For this review, take the finished solid that the model builds, in its own axes (mm). Face numbers are marked on the shaded views. A direction names the side the tool comes from. Give positions to 0.01 mm unless a question says otherwise; leave off trailing zeros. Order: outer loops, then holes, each group sorted by start corner. A loop starts at its lowest first (then second) coordinate and runs counter-clockwise, first axis right, second up. Notation, with made-up numbers: (39, 5) - (66, 5) arc R16 cw to (66, 26) - close; hole circle Ø2 at (-27.5, -30.5). An arc over 180 degrees is marked (long way). One line per item, written item: value.
```python
from build123d import *

# Parameters (mm, degrees)
SKETCH1_R           = 3.5
SKETCH1_R_2         = 4.5
BOSS_EXTRUDE1_DEPTH = 5
SKETCH2_R           = 8.75
SKETCH2_R_2         = 3.5
SKETCH2_R_3         = 4.5
BOSS_EXTRUDE2_DEPTH = 5


with BuildPart() as part:
    # Sketch1 → Boss-Extrude1 (new body)
    with BuildSketch(Plane.XY):
        with BuildLine():
            Line((-12.068862554, -6.04917818), (-9.828426191, -10.519127274))
            ThreePointArc((-9.828426191, -10.519127274), (-9.022245749, -17.239185417), (-12.680657026, -22.933492686))
            Line((-12.680657026, -22.933492686), (-18.627117662, -27.496435605))
            ThreePointArc((-18.627117662, -27.496435605), (-21.193595331, -47.96861112), (-0.691265287, -50.281886009))
            Line((-0.691265287, -50.281886009), (7.089345754, -44))
            Line((7.089345754, -44), (46.481655875, -37.054072893))
            Line((46.481655875, -37.054072893), (39.535728768, 2.338237227))
            ThreePointArc((39.535728768, 2.338237227), (23.15933572, 3.004735652), (8.554710295, 10.443511467))
            ThreePointArc((8.554710295, 10.443511467), (-8.431460103, 10.543267071), (-12.068862554, -6.04917818))
        make_face()
        Circle(SKETCH1_R, mode=Mode.SUBTRACT)
        with Locations((-9.8, -39)):
            Circle(SKETCH1_R_2, mode=Mode.SUBTRACT)
    extrude(amount=-BOSS_EXTRUDE1_DEPTH)

    # Sketch2 → Boss-Extrude2 (add)
    # profile 1 of 2: a face of its own
    with BuildSketch(Plane(origin=(0, 0, -5), x_dir=(-1, 0, 0), z_dir=(0, 0, -1))):
        with Locations(Location((0, 0, 0), (0, 0, 180))):
            Circle(SKETCH2_R)
        with Locations(Location((0, 0, 0), (0, 0, 180))):
            Circle(SKETCH2_R_2, mode=Mode.SUBTRACT)
    # profile 2 of 2: a face of its own
    with BuildSketch(Plane(origin=(0, 0, -5), x_dir=(-1, 0, 0), z_dir=(0, 0, -1))):
        with Locations(Location((9.8, -39, 0), (0, 0, 180))):
            Circle(SKETCH2_R)
        with Locations(Location((9.8, -39, 0), (0, 0, 180))):
            Circle(SKETCH2_R_3, mode=Mode.SUBTRACT)
    extrude(amount=BOSS_EXTRUDE2_DEPTH)


solid = part.part
```
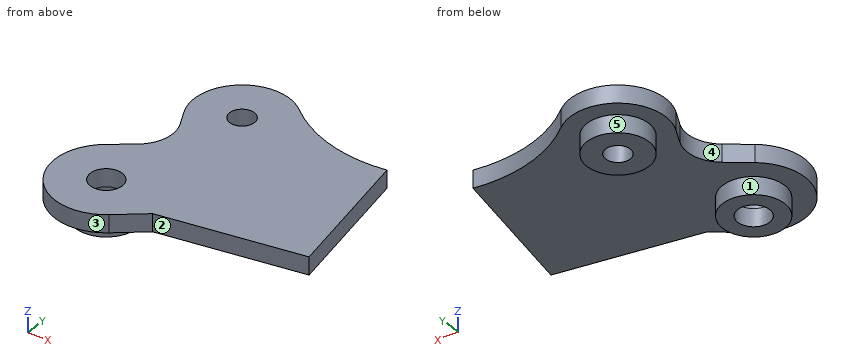
(1) Machinability: for the marked faces 4 and 5, which of the approach directions +Z, -Z, +X, -X, +Y, -Y give a long, thin tool a straight path to every point of the face, cutting with its end or side? Answer none if there is none.
Answers below:
face 4: +Z, -Z, -X
face 5: -Z
(2) Take a section at C-C (y = -5). Write out the cut boundary in (x, z), then the cut area to 3 significant figures.
Answers below:
outline: (-12.54, -5) - (-7.18, -5) - (-7.18, -10) - (7.18, -10) - (7.18, -5) - (40.83, -5) - (40.83, 0) - (-12.54, 0) - close
area: 339 mm^2
(3) Wall thickness on line 1 (X direction, y = -39, z = -8.9); line 2 (Y direction, x = 0, z = -6.8); line 3 (Z direction, x = 17.5, y = -38.5): over which ranges is each line inside the solid? List them lowest first. Write a range as from..to.
Answers below:
line 1: x = -18.55..-14.3, -5.3..-1.05
line 2: y = -8.75..-3.5, 3.5..8.75
line 3: z = -5..0
(4) Take a section at A-A (y = -39). Write out the cut boundary in (x, z), then the cut area to 3 significant figures.
Answers below:
outline: (-24.3, -5) - (-18.55, -5) - (-18.55, -10) - (-14.3, -10) - (-14.3, 0) - (-24.3, 0) - close; (-5.3, -10) - (-1.05, -10) - (-1.05, -5) - (35.45, -5) - (35.45, 0) - (-5.3, 0) - close
area: 296 mm^2
(5) Take a section at D-D (x = -4.5). Write out the cut boundary in (y, z), then the cut area to 3 significant figures.
Answers below:
outline: (-52.5, -5) - (-45.96, -5) - (-45.96, -10) - (-32.04, -10) - (-32.04, -5) - (-7.5, -5) - (-7.5, -10) - (7.5, -10) - (7.5, -5) - (12.73, -5) - (12.73, 0) - (-52.5, 0) - close
area: 471 mm^2
(6) For P1, Ø6, axis at x = 17.5, z = -7, coming from the -Y side; P2, Ø1, axis at x = 8.5, z = -2, coming from the -Y side; P3, Ø3, axis at y = 1, z = -2.5, coming from the +X side, all flat-tipped, find the tip position at first contact; note any pin that passes through.
Answers below:
P1: stops at y = -42.56
P2: stops at y = -43.84
P3: stops at x = 40.04
(7) Take a section at B-B (z = -6.25). Write out the cut boundary in (x, y), then the cut area to 3 significant figures.
Answers below:
outline: circle Ø17.5 at (-9.8, -39); circle Ø17.5 at (0, 0); hole circle Ø9 at (-9.8, -39); hole circle Ø7 at (0, 0)
area: 379 mm^2
(8) Draft analysis for pull direction Y (two halves, no side actions). For the marked faces 1, 2 and 3, state which applies: pulls with the +Y half, pulls with the -Y half, needs draft (parallel to the pull), parting line crosses it, or undercut.
Answers below:
face 1: undercut
face 2: pulls with the -Y half
face 3: parting line crosses it
